Work out the finished part from the listing and answer in its coordinate system (mm). Give positions to 0.01 mm unless a question says otherwise; leave off trailing zeros. Order: outer loops, then holes, each group sorted by start corner. A loop starts at its lowest first (then second) coordinate and runs counter-clockwise, first axis right, second up. Notation, with made-up numbers: (6, -23.75) -> (48, -23.75) arc R21 ccw to (48, -6.75) -> close; hole circle Ø9 at (-38, 45). An arc over 180 degrees is marked (long way). Answer as CSV lines item,"result". Start each with the question number.
1. A cutting plane is placed at A-A (y = 0). State how many separate pieces and enclosed holes the cut face has, then the cut area to 3 significant figures.
2. For a pull along Y with two mould halves and no side action, classify faces 1 (the flat face through (-44.475, 5.634, 0.986)), 2 (the cylindrical face through (51.8, -0.1, 1)), 3 (the cylindrical face through (0.228, -49.535, 0.986)), 4 (the flat face through (-5.634, -44.475, 0.986)) as released by +Y, released by -Y, zero draft, split by the parting line, or undercut.
3. A cutting plane is placed at D-D (y = -44). Give the vertices of the cut face in (x, z).
4. Flat-ended cylindrical pins translate along their axes: pin 1 (1 mm diameter, centred on x = -23, z = 1, fed in from +Y); pin 2 (1 mm diameter, centred on x = -33, y = -25, fed in from +Z). Find the tip coordinate at first contact, or state that the pin passes through.
5. Find the intervals of material crossed by L1, parallel to Y at x = 0, z = 1.45; L2, parallel to Y at x = -0.5, z = 1.6; L3, parallel to Y at x = -47, z = 1.6, in increasing order.
from build123d import *

# Parameters (mm, degrees)
SKETCH1_R           = 40.5
SKETCH1_R_2         = 35
BOSS_EXTRUDE1_DEPTH = 2
SKETCH2_R           = 1.75
BOSS_EXTRUDE2_DEPTH = 2
CIRPATTERN1_COUNT   = 4
CHAMFER1_SIZE       = 2


with BuildPart() as part:
    # Sketch1 → Boss-Extrude1 (new body)
    with BuildSketch(Plane.XY):
        Circle(SKETCH1_R)
        Circle(SKETCH1_R_2, mode=Mode.SUBTRACT)
    extrude(amount=BOSS_EXTRUDE1_DEPTH)

    # Sketch2 → Boss-Extrude2 (add)
    with BuildSketch(Plane.XY):
        with BuildLine():
            Line((7.5, 39.799497484), (3.715004122, 49.282313849))
            ThreePointArc((3.715004122, 49.282313849), (0, 51.799497484), (-3.715004122, 49.282313849))
            Line((-3.715004122, 49.282313849), (-7.5, 39.799497484))
            ThreePointArc((-7.5, 39.799497484), (0, 40.5), (7.5, 39.799497484))
        make_face()
        with Locations((0, 47.799497484)):
            Circle(SKETCH2_R, mode=Mode.SUBTRACT)
    boss_extrude2 = extrude(amount=BOSS_EXTRUDE2_DEPTH)

    # CirPattern1: Boss-Extrude2 ×4 about axis
    cirpattern1_axis = Axis((0, 0, 0), (0, 0, 1))
    for i in range(1, CIRPATTERN1_COUNT):
        add(boss_extrude2.rotate(cirpattern1_axis, i * 360 / CIRPATTERN1_COUNT))

    # Chamfer1
    chamfer1_edges = [part.edges().sort_by_distance(p)[0] for p in [
        (-35, 0, 2),
    ]]
    chamfer(chamfer1_edges, length=CHAMFER1_SIZE - 0.0001)  # a hair under: the kernel refuses the full size


solid = part.part
Answer sheet:
1,separate pieces,"4"
1,enclosed holes,"0"
1,area,"49.2 mm^2"
2,face 1,"released by +Y"
2,face 2,"split by the parting line"
2,face 3,"undercut"
2,face 4,"released by -Y"
3,outline,"(-5.82, 0) -> (5.82, 0) -> (5.82, 2) -> (-5.82, 2) -> close"
4,pin 1,"stops at y = 33.67"
4,pin 2,"passes through"
5,L1,"y = -51.8 to -49.55, -46.05 to -36.45, 36.45 to 46.05, 49.55 to 51.8"
5,L2,"y = -51.77 to -49.48, -46.12 to -36.6, 36.6 to 46.12, 49.48 to 51.77"
5,L3,"y = -4.63 to -1.56, 1.56 to 4.63"
